from build123d import *

# Parameters (mm, degrees)
BASE_SKETCH_R = 7.6
BASE_DEPTH    = 24.4


with BuildPart() as part:
    # Base Sketch → Base (new body)
    with BuildSketch(Plane.XY):
        with BuildLine():
            ThreePointArc((30, 13.049209956), (14.080181926, 9.934954429), (0.706182938, 0.75479397))
            ThreePointArc((0.706182938, 0.75479397), (0.674336237, 0.449442107), (0.96247377, 0.34346695))
            ThreePointArc((0.96247377, 0.34346695), (10.955807445, 0.032866395), (18.534024513, -6.488929117))
            ThreePointArc((18.534024513, -6.488929117), (41.11144962, -6.605033659), (30, 13.049209956))
        make_face()
        with Locations((28.406836056, -1.449568901)):
            Circle(BASE_SKETCH_R, mode=Mode.SUBTRACT)
    extrude(amount=-BASE_DEPTH)


solid = part.part
The model under review builds one solid part; all positions refer to its coordinate system, in mm. Round coordinates to 2 decimals unless told otherwise and drop trailing zeros. Write each loop counter-clockwise with the first axis right and the second up, starting at its lowest first coordinate (ties: lowest second). Pieces come first, ordered by that corner, then holes. Notation, with made-up numbers: M 29.25,3 L 58.25,3 A15 ccw 58.25,10 Z; hole C 49,61 d1. An arc over 180 degrees is marked long. Use a Markdown table: item, result. Add a question column.
Q1. To check wall thickness, follow line 1 (X direction, y = -1.25, z = -8.5); line 2 (X direction, y = 4.25, z = -2.5); line 3 (Y direction, x = 6.5, z = -7). State the ranges of each line that lie inside material, in increasing order.
Q2. The part is to be moulded in two halves that separate along X. For faces 1 (the face through (22.376, -6.074, -12.029)), 2 (the face through (40.913, -6.932, -12.029)), 3 (the face through (26, 6, -24.4)), say which applies: pulls with the +X half, pulls with the -X half, needs draft (parallel to the pull), parting line crosses it, or undercut.
Q3. We need section D-D, the plane x = 12. State the section outline as (y, z) points, plus the area to 3 significant figures.
Q4. Insertion check: pin 1 (10 mm diameter, centred on y = -7, z = -13, fed in from -X); pin 2 (2 mm diameter, centred on x = 33.5, z = -13.5, fed in from +Y); pin 3 (1 mm diameter, centred on x = 12.5, z = -9, fed in from -Y). Each pin has a flat end and moves straight along its axis. Give the tip position at first contact, or say it passes through.
Q5. We need section A-A, the plane x = 21.5. State the section outline as (y, z) points, plus the area to 3 significant figures.
Q6. We need section B-B, the plane y = 1.5. State the section outline as (x, z) points.
Q7. We need section C-C, the plane z = -18. State the section outline as (x, y) points, plus the area to 3 significant figures.
Findings below:
| question | item | result |
|---|---|---|
| 1 | line 1 | x = 13.51 to 20.81, 36 to 42.85 |
| 1 | line 2 | x = 4.53 to 23.38, 33.43 to 42.19 |
| 1 | line 3 | y = 1.02 to 5.74 |
| 2 | face 1 | undercut |
| 2 | face 2 | parting line crosses it |
| 2 | face 3 | needs draft |
| 3 | outline | M -0.42,-24.4 L 8.99,-24.4 L 8.99,0 L -0.42,0 Z |
| 3 | area | 230 mm² |
| 4 | pin 1 | stops at x = 14.59 |
| 4 | pin 2 | stops at y = 12.78 |
| 4 | pin 3 | stops at y = -0.95 |
| 5 | outline | M -10.02,-24.4 L -4.62,-24.4 L -4.62,0 L -10.02,0 Z; M 1.72,-24.4 L 12.23,-24.4 L 12.23,0 L 1.72,0 Z |
| 5 | area | 388 mm² |
| 6 | outline | M 1.44,-24.4 L 21.4,-24.4 L 21.4,0 L 1.44,0 Z; M 35.41,-24.4 L 42.82,-24.4 L 42.82,0 L 35.41,0 Z |
| 7 | outline | M 0.71,0.75 A0.25 ccw 0.96,0.34 A15 cw 18.53,-6.49 A13.05 ccw long 30,13.05 A40 ccw Z; hole C 28.41,-1.45 d15.2 |
| 7 | area | 494 mm² |
